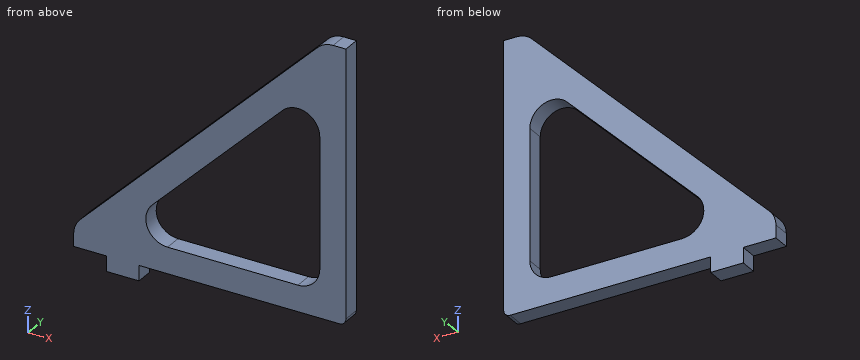
```python
from build123d import *

# Parameters (mm, degrees)
F1_DEPTH = 8


with BuildPart() as f1:
    # F0 (on Front) → F1 (new body)
    with BuildSketch(Plane.XZ):
        with BuildLine():
            ThreePointArc((-3, 0), (-0.87868, 0.87868), (0, 3))
            Line((0, 3), (0, 125))
            Line((0, 125), (-5.857864, 125))
            ThreePointArc((-5.857864, 125), (-9.684699, 124.238795), (-12.928932, 122.071068))
            Line((-12.928932, 122.071068), (-122.071068, 12.928932))
            ThreePointArc((-122.071068, 12.928932), (-124.238795, 9.684699), (-125, 5.857864))
            Line((-125, 5.857864), (-125, 0))
            Line((-125, 0), (-110, 0))
            Line((-110, 0), (-110, -7))
            Line((-110, -7), (-95, -7))
            Line((-95, -7), (-95, 0))
            Line((-95, 0), (-3, 0))
        make_face()
        with BuildLine():
            ThreePointArc((-29.071068, 88.958369), (-18.173166, 91.126097), (-12, 81.887302))
            Line((-12, 81.887302), (-12, 22))
            ThreePointArc((-12, 22), (-14.928932, 14.928932), (-22, 12))
            Line((-22, 12), (-81.887302, 12))
            ThreePointArc((-81.887302, 12), (-91.126097, 18.173166), (-88.958369, 29.071068))
            Line((-88.958369, 29.071068), (-29.071068, 88.958369))
        make_face(mode=Mode.SUBTRACT)
    extrude(amount=F1_DEPTH)


solid = f1.part
```
Check sheet for the modelled part. Datum: model origin and axes. Units: mm. Coordinates: 2 decimals unless noted, no trailing zeros. Loops run counter-clockwise (first coordinate to the right, second up) from the corner with the lowest first, then second, coordinate; pieces in that order, holes last.
1) Sectioned sample at B-B (y = -6). Record the boundary of the cut face in (x, z), and give its area (3 significant figures).
2) Material ranges on probe 1 along Z at (x, y) = (-87, -4.5); probe 2 along X at (y, z) = (-3, 78.5); probe 3 along Z at (x, y) = (-6, -2), recorded low to high.
3) Gauge pin test, flat ends, axial feed: pin 1 (4 mm diameter, centred on x = -27, y = -5.5, fed in from -Z); pin 2 (1.5 mm diameter, centred on y = -5, z = 6.5, fed in from -X). Record the tip position at first contact, or that the pin passes through.
4) Sectioned sample at C-C (z = 58.5). Record the boundary of the cut face in (x, y).
5) Sectioned sample at A-A (x = -76). Record the boundary of the cut face in (y, z), and give its area (3 significant figures).
6) Sectioned sample at D-D (x = -111.5). Record the boundary of the cut face in (y, z), and give its area (3 significant figures).
Check sheet entries:
1. outline: (-125, 0) - (-110, 0) - (-110, -7) - (-95, -7) - (-95, 0) - (-3, 0) arc R3 ccw to (0, 3) - (0, 125) - (-5.86, 125) arc R10 ccw to (-12.93, 122.07) - (-122.07, 12.93) arc R10 ccw to (-125, 5.86) - close; hole (-88.96, 29.07) arc R10 ccw to (-81.89, 12) - (-22, 12) arc R10 ccw to (-12, 22) - (-12, 81.89) arc R10 ccw to (-29.07, 88.96) - close
1. area: 4,960 mm2
2. probe 1: z = 0 to 13.41, 31.03 to 48
2. probe 2: x = -56.5 to -39.53, -12 to 0
2. probe 3: z = 0 to 125
3. pin 1: stops at z = 0
3. pin 2: stops at x = -125
4. outline: (-76.5, -8) - (-59.53, -8) - (-59.53, 0) - (-76.5, 0) - close; (-12, -8) - (0, -8) - (0, 0) - (-12, 0) - close
5. outline: (-8, 0) - (0, 0) - (0, 12) - (-8, 12) - close; (-8, 42.03) - (0, 42.03) - (0, 59) - (-8, 59) - close
5. area: 232 mm2
6. outline: (-8, 0) - (0, 0) - (0, 23.5) - (-8, 23.5) - close
6. area: 188 mm2
